Read the model definition and answer for the solid it produces. Units are mm, in the model's axes. A direction names the side the tool comes from. Coordinates: 2 decimals unless noted, no trailing zeros. Loops run counter-clockwise (first coordinate to the right, second up) from the corner with the lowest first, then second, coordinate; pieces in that order, holes last. Notation, with made-up numbers: M 4.5,-39.5 L 42.5,-39.5 A26 ccw 42.5,-20.5 Z; hole C 30,4.25 d4. An arc over 180 degrees is marked long. One line per item, written item: value. Start each with the question number.
```python
from build123d import *

# Parameters (mm, degrees)
SKETCH1_W           = 143.8
SKETCH1_H           = 41.8
SKETCH1_R           = 1.5875
BOSS_EXTRUDE1_DEPTH = 3
SKETCH4_W           = 10
SKETCH4_H           = 8
BOSS_EXTRUDE3_DEPTH = 10
CHAMFER2_SIZE       = 5
SKETCH5_R           = 2.2
CUT_EXTRUDE2_DEPTH  = 5.2
CUT_EXTRUDE3_DEPTH  = 10
CHAMFER3_SIZE       = 1
SKETCH8_W           = 5
SKETCH8_H           = 20
CUT_EXTRUDE4_DEPTH  = 10
FILLET1_R           = 2


with BuildPart() as part:
    # Sketch1 → Boss-Extrude1 (new body)
    with BuildSketch(Plane(origin=(0, 0, 0), x_dir=(1, 0, 0), z_dir=(0, 1, 0))):
        Rectangle(SKETCH1_W, SKETCH1_H)
        with Locations(Location((-57.2125, 15.621, 0), (0, 0, 270))):
            Circle(SKETCH1_R, mode=Mode.SUBTRACT)
        with Locations(Location((-44.5125, 15.621, 0), (0, 0, 270))):
            Circle(SKETCH1_R, mode=Mode.SUBTRACT)
        with Locations(Location((-25.4625, 15.621, 0), (0, 0, 270))):
            Circle(SKETCH1_R, mode=Mode.SUBTRACT)
        with Locations(Location((-25.4625, -15.621, 0), (0, 0, 270))):
            Circle(SKETCH1_R, mode=Mode.SUBTRACT)
        with Locations(Location((-44.5125, -15.621, 0), (0, 0, 270))):
            Circle(SKETCH1_R, mode=Mode.SUBTRACT)
        with Locations(Location((-57.2125, -15.621, 0), (0, 0, 270))):
            Circle(SKETCH1_R, mode=Mode.SUBTRACT)
        with Locations(Location((44.5125, -15.621, 0), (0, 0, 90))):
            Circle(SKETCH1_R, mode=Mode.SUBTRACT)
        with Locations(Location((25.4625, -15.621, 0), (0, 0, 90))):
            Circle(SKETCH1_R, mode=Mode.SUBTRACT)
        with Locations(Location((25.4625, 15.621, 0), (0, 0, 90))):
            Circle(SKETCH1_R, mode=Mode.SUBTRACT)
        with Locations(Location((44.5125, 15.621, 0), (0, 0, 90))):
            Circle(SKETCH1_R, mode=Mode.SUBTRACT)
        with Locations(Location((57.2125, 15.621, 0), (0, 0, 90))):
            Circle(SKETCH1_R, mode=Mode.SUBTRACT)
        with Locations(Location((57.2125, -15.621, 0), (0, 0, 90))):
            Circle(SKETCH1_R, mode=Mode.SUBTRACT)
    extrude(amount=BOSS_EXTRUDE1_DEPTH)

    # Sketch4 → Boss-Extrude3 (add)
    with BuildSketch(Plane(origin=(0, 3, 0), x_dir=(1, 0, 0), z_dir=(0, 1, 0))):
        with Locations((-34.9875, 16.9)):
            Rectangle(SKETCH4_W, SKETCH4_H)
        with Locations((34.9875, 16.9)):
            Rectangle(SKETCH4_W, SKETCH4_H)
    extrude(amount=BOSS_EXTRUDE3_DEPTH)

    # Chamfer2
    chamfer2_edges = [part.edges().sort_by_distance(p)[0] for p in [
        (-34.9875, 3, -12.9),
        (34.9875, 3, -12.9),
    ]]
    chamfer(chamfer2_edges, length=CHAMFER2_SIZE)

    # Sketch5 → Cut-Extrude2 (cut)
    with BuildSketch(Plane(origin=(0, 0, -20.9), x_dir=(-1, 0, 0), z_dir=(0, 0, -1))):
        with Locations((-34.9875, 6.5)):
            Circle(SKETCH5_R)
        with Locations((34.9875, 6.5)):
            Circle(SKETCH5_R)
    extrude(amount=-CUT_EXTRUDE2_DEPTH, mode=Mode.SUBTRACT)

    # Sketch7 → Cut-Extrude3 (cut)
    with BuildSketch(Plane(origin=(0, 3, 0), x_dir=(1, 0, 0), z_dir=(0, 1, 0))):
        with BuildLine():
            Line((-56.4625, 13.921), (-57.9625, 13.921))
            ThreePointArc((-57.9625, 13.921), (-59.6625, 15.621), (-57.9625, 17.321))
            Line((-57.9625, 17.321), (-56.4625, 17.321))
            ThreePointArc((-56.4625, 17.321), (-54.7625, 15.621), (-56.4625, 13.921))
        make_face()
        with BuildLine():
            Line((-43.7625, 13.921), (-45.2625, 13.921))
            ThreePointArc((-45.2625, 13.921), (-46.9625, 15.621), (-45.2625, 17.321))
            Line((-45.2625, 17.321), (-43.7625, 17.321))
            ThreePointArc((-43.7625, 17.321), (-42.0625, 15.621), (-43.7625, 13.921))
        make_face()
        with BuildLine():
            Line((-26.2125, 17.321), (-24.7125, 17.321))
            ThreePointArc((-24.7125, 17.321), (-23.0125, 15.621), (-24.7125, 13.921))
            Line((-24.7125, 13.921), (-26.2125, 13.921))
            ThreePointArc((-26.2125, 13.921), (-27.9125, 15.621), (-26.2125, 17.321))
        make_face()
        with BuildLine():
            Line((-43.7625, -17.321), (-45.2625, -17.321))
            ThreePointArc((-45.2625, -17.321), (-46.9625, -15.621), (-45.2625, -13.921))
            Line((-45.2625, -13.921), (-43.7625, -13.921))
            ThreePointArc((-43.7625, -13.921), (-42.0625, -15.621), (-43.7625, -17.321))
        make_face()
        with BuildLine():
            Line((-57.9625, -13.921), (-56.4625, -13.921))
            ThreePointArc((-56.4625, -13.921), (-54.7625, -15.621), (-56.4625, -17.321))
            Line((-56.4625, -17.321), (-57.9625, -17.321))
            ThreePointArc((-57.9625, -17.321), (-59.6625, -15.621), (-57.9625, -13.921))
        make_face()
        with BuildLine():
            Line((-24.7125, -17.321), (-26.2125, -17.321))
            ThreePointArc((-26.2125, -17.321), (-27.9125, -15.621), (-26.2125, -13.921))
            Line((-26.2125, -13.921), (-24.7125, -13.921))
            ThreePointArc((-24.7125, -13.921), (-23.0125, -15.621), (-24.7125, -17.321))
        make_face()
        with BuildLine():
            Line((56.4625, -13.921), (57.9625, -13.921))
            ThreePointArc((57.9625, -13.921), (59.6625, -15.621), (57.9625, -17.321))
            Line((57.9625, -17.321), (56.4625, -17.321))
            ThreePointArc((56.4625, -17.321), (54.7625, -15.621), (56.4625, -13.921))
        make_face()
        with BuildLine():
            Line((45.2625, -17.321), (43.7625, -17.321))
            ThreePointArc((43.7625, -17.321), (42.0625, -15.621), (43.7625, -13.921))
            Line((43.7625, -13.921), (45.2625, -13.921))
            ThreePointArc((45.2625, -13.921), (46.9625, -15.621), (45.2625, -17.321))
        make_face()
        with BuildLine():
            Line((24.7125, -13.921), (26.2125, -13.921))
            ThreePointArc((26.2125, -13.921), (27.9125, -15.621), (26.2125, -17.321))
            Line((26.2125, -17.321), (24.7125, -17.321))
            ThreePointArc((24.7125, -17.321), (23.0125, -15.621), (24.7125, -13.921))
        make_face()
        with BuildLine():
            Line((56.4625, 17.321), (57.9625, 17.321))
            ThreePointArc((57.9625, 17.321), (59.6625, 15.621), (57.9625, 13.921))
            Line((57.9625, 13.921), (56.4625, 13.921))
            ThreePointArc((56.4625, 13.921), (54.7625, 15.621), (56.4625, 17.321))
        make_face()
        with BuildLine():
            Line((43.7625, 17.321), (45.2625, 17.321))
            ThreePointArc((45.2625, 17.321), (46.9625, 15.621), (45.2625, 13.921))
            Line((45.2625, 13.921), (43.7625, 13.921))
            ThreePointArc((43.7625, 13.921), (42.0625, 15.621), (43.7625, 17.321))
        make_face()
        with BuildLine():
            Line((26.2125, 13.921), (24.7125, 13.921))
            ThreePointArc((24.7125, 13.921), (23.0125, 15.621), (24.7125, 17.321))
            Line((24.7125, 17.321), (26.2125, 17.321))
            ThreePointArc((26.2125, 17.321), (27.9125, 15.621), (26.2125, 13.921))
        make_face()
    extrude(amount=-CUT_EXTRUDE3_DEPTH, mode=Mode.SUBTRACT)

    # Chamfer3
    chamfer3_edges = [part.edges().sort_by_distance(p)[0] for p in [
        (-23.0125, 3, 15.621),
        (-25.4625, 3, 13.921),
        (-27.9125, 3, 15.621),
        (-25.4625, 3, 17.321),
        (54.7625, 3, 15.621),
        (57.2125, 3, 17.321),
        (59.6625, 3, 15.621),
        (57.2125, 3, 13.921),
        (46.9625, 3, 15.621),
        (44.5125, 3, 13.921),
        (42.0625, 3, 15.621),
        (44.5125, 3, 17.321),
        (23.0125, 3, 15.621),
        (25.4625, 3, 17.321),
        (27.9125, 3, 15.621),
        (25.4625, 3, 13.921),
        (-59.6625, 3, 15.621),
        (-57.2125, 3, 17.321),
        (-54.7625, 3, 15.621),
        (-57.2125, 3, 13.921),
        (-42.0625, 3, 15.621),
        (-44.5125, 3, 13.921),
        (-46.9625, 3, 15.621),
        (-44.5125, 3, 17.321),
        (-27.9125, 3, -15.621),
        (-25.4625, 3, -13.921),
        (-23.0125, 3, -15.621),
        (-25.4625, 3, -17.321),
        (-42.0625, 3, -15.621),
        (-44.5125, 3, -17.321),
        (-46.9625, 3, -15.621),
        (-44.5125, 3, -13.921),
        (54.7625, 3, -15.621),
        (57.2125, 3, -13.921),
        (59.6625, 3, -15.621),
        (57.2125, 3, -17.321),
        (42.0625, 3, -15.621),
        (44.5125, 3, -13.921),
        (46.9625, 3, -15.621),
        (44.5125, 3, -17.321),
        (27.9125, 3, -15.621),
        (25.4625, 3, -17.321),
        (23.0125, 3, -15.621),
        (25.4625, 3, -13.921),
        (-54.7625, 3, -15.621),
        (-57.2125, 3, -17.321),
        (-59.6625, 3, -15.621),
        (-57.2125, 3, -13.921),
    ]]
    chamfer(chamfer3_edges, length=CHAMFER3_SIZE)

    # Sketch8 → Cut-Extrude4 (cut)
    with BuildSketch(Plane(origin=(0, 3, 0), x_dir=(1, 0, 0), z_dir=(0, 1, 0))):
        with Locations((12.326083865, 0)):
            Rectangle(SKETCH8_W, SKETCH8_H)
        with Locations((-12.326083865, 0)):
            Rectangle(SKETCH8_W, SKETCH8_H)
    extrude(amount=-CUT_EXTRUDE4_DEPTH, mode=Mode.SUBTRACT)

    # Fillet1
    fillet1_edges = [part.edges().sort_by_distance(p)[0] for p in [
        (-9.826083865, 1.5, -10),
        (-9.826083865, 1.5, 10),
        (-14.826083865, 1.5, 10),
        (-14.826083865, 1.5, -10),
        (14.826083865, 1.5, -10),
        (14.826083865, 1.5, 10),
        (9.826083865, 1.5, 10),
        (9.826083865, 1.5, -10),
    ]]
    fillet(fillet1_edges, radius=FILLET1_R)


solid = part.part
```
1) Section B-B (z = 1) is taken. Determine the outline of the cut face in (x, y), then the cut area to 3 significant figures.
2) Section A-A (y = 6.5) is taken. Determine the outline of the cut face in (x, z), then the cut area to 3 significant figures.
3) Consider line 1 along X through (y, z) = (6, -13.5); line 2 along X through (y, z) = (0.5, -6.5); line 3 along X through (y, z) = (7.5, -18.5). Determine where each line is inside the solid, lowest interval first.
4) Flat-ended cylindrical pins translate along their axes: pin 1 (5 mm diameter, centred on y = 10, z = -13, fed in from +X); pin 2 (5 mm diameter, centred on y = 6, z = -17, fed in from -X); pin 3 (1.5 mm diameter, centred on x = 33.5, y = 10.5, fed in from +Z). Find the tip coordinate at first contact, or state that the pin passes through.
5) For a pull along X with two mould halves and no side action, classify faces 1 (the face through (22.853, 2.16, 15.662)), 2 (the face through (35, 13, -17)) as released by +X, released by -X, zero draft, split by the parting line, or undercut.
6) Section C-C (x = 7) is taken. Determine the outline of the cut face in (y, z), then the cut area to 3 significant figures.
7) A tool of negligible diameter and unlimited length cuts with its end or side. For faces 3 (the face through (-47.12, 2.16, 15.66)), 4 (the face through (35, 7, -15.7)), 5 (the face through (-29.987, 7, -16)), from which of +Z, -Z, +X, -X, +Y, -Y can it reach the whole face along a straight path? Write none if from no direction.
Results found:
1. outline: M -71.9,0 L -14.83,0 L -14.83,3 L -71.9,3 Z; M -9.83,0 L 9.83,0 L 9.83,3 L -9.83,3 Z; M 14.83,0 L 71.9,0 L 71.9,3 L 14.83,3 Z
1. area: 401 mm²
2. outline: M -39.99,-20.9 L -37.19,-20.9 L -37.19,-15.7 L -32.79,-15.7 L -32.79,-20.9 L -29.99,-20.9 L -29.99,-11.4 L -39.99,-11.4 Z; M 29.99,-20.9 L 32.79,-20.9 L 32.79,-15.7 L 37.19,-15.7 L 37.19,-20.9 L 39.99,-20.9 L 39.99,-11.4 L 29.99,-11.4 Z
2. area: 144 mm²
3. line 1: x = -39.99 to -29.99, 29.99 to 39.99
3. line 2: x = -71.9 to -14.83, -9.83 to 9.83, 14.83 to 71.9
3. line 3: x = -39.99 to -36.95, -33.03 to -29.99, 29.99 to 33.03, 36.95 to 39.99
4. pin 1: stops at x = 39.99
4. pin 2: stops at x = -39.99
4. pin 3: stops at z = -12.9
5. face 1: undercut
5. face 2: zero draft
6. outline: M 0,-20.9 L 3,-20.9 L 3,20.9 L 0,20.9 Z
6. area: 125 mm²
7. face 3: +Y
7. face 4: -Z
7. face 5: +Z, -Z, +Y
